from build123d import *

# Parameters (mm, degrees)
F0_R     = 12.7
F0_R_2   = 6.35
F1_DEPTH = 25.4
F2_R     = 5.08


with BuildPart() as f1:
    # F0 (on Front) → F1 (new body)
    with BuildSketch(Plane.XZ):
        Polygon((-25.4, 0), (0, 0), (25.4, 0), (25.4, 76.2), (63.5, 76.2), (63.5, 127), (-63.5, 127), (-63.5, 76.2), (-25.4, 76.2), align=None)
        with Locations((-38.1, 101.6)):
            Circle(F0_R, mode=Mode.SUBTRACT)
        with Locations((38.1, 101.6)):
            Circle(F0_R, mode=Mode.SUBTRACT)
        Polygon((25.4, 0), (0, 0), (-25.4, 0), (-25.4, -38.1), (-101.6, -38.1), (-101.6, -101.6), (101.6, -101.6), (101.6, -38.1), (25.4, -38.1), align=None)
        with Locations((-76.2, -69.85)):
            Circle(F0_R_2, mode=Mode.SUBTRACT)
        with Locations((-38.1, -69.85)):
            Circle(F0_R_2, mode=Mode.SUBTRACT)
        with Locations((38.1, -69.85)):
            Circle(F0_R_2, mode=Mode.SUBTRACT)
        with Locations((76.2, -69.85)):
            Circle(F0_R_2, mode=Mode.SUBTRACT)
    extrude(amount=F1_DEPTH)

    # F2
    f2_edges = [f1.edges().sort_by_distance(p)[0] for p in [
        (-25.4, -12.7, 76.2),
        (-25.4, -12.7, -38.1),
        (25.4, -12.7, -38.1),
        (25.4, -12.7, 76.2),
    ]]
    fillet(f2_edges, radius=F2_R)


solid = f1.part
The listing builds one solid part. Answer for the finished solid, in the listing's coordinates (mm). A direction names the side the tool comes from. Coordinates: 2 decimals unless noted, no trailing zeros. Write each loop counter-clockwise with the first axis right and the second up, starting at its lowest first coordinate (ties: lowest second). Pieces come first, ordered by that corner, then holes. Notation, with made-up numbers: (23, -11) -> (42, -11) arc R9 cw to (42, -5) -> close; hole circle Ø4 at (18, 6.25). An arc over 180 degrees is marked (long way). One line per question, with ' | ' between items.
1. For a pull along Z with two mould halves and no side action, classify faces 4 (the flat face through (-1, -13, -101.6)), 5 (the cylindrical face through (-39.753, -12.522, 114.192)), 6 (the flat face through (-1, -25.4, -11)) as released by +Z, released by -Z, zero draft, split by the parting line, or undercut.
Verdict:
face 4: released by -Z | face 5: undercut | face 6: zero draft
2. Section D-D (y = -11.5) is taken. Determine the outline of the cut face in (x, z).
Verdict:
outline: (-101.6, -101.6) -> (101.6, -101.6) -> (101.6, -38.1) -> (30.48, -38.1) arc R5.08 cw to (25.4, -33.02) -> (25.4, 71.12) arc R5.08 cw to (30.48, 76.2) -> (63.5, 76.2) -> (63.5, 127) -> (-63.5, 127) -> (-63.5, 76.2) -> (-30.48, 76.2) arc R5.08 cw to (-25.4, 71.12) -> (-25.4, -33.02) arc R5.08 cw to (-30.48, -38.1) -> (-101.6, -38.1) -> close; hole circle Ø12.7 at (-76.2, -69.85); hole circle Ø25.4 at (-38.1, 101.6); hole circle Ø12.7 at (-38.1, -69.85); hole circle Ø25.4 at (38.1, 101.6); hole circle Ø12.7 at (38.1, -69.85); hole circle Ø12.7 at (76.2, -69.85)
3. Given pin 1 Ø7.5 at (y, z) = (-16.5, 17.5) entering from +X; pin 2 Ø1 at (y, z) = (-15.5, 104) entering from +X; pin 3 Ø10 at (y, z) = (-5.5, 54.5) entering from -X, each flat-ended and moving along its own axis, determine where each tip first touches the part or whether it passes through.
Verdict:
pin 1: stops at x = 25.4 | pin 2: stops at x = 63.5 | pin 3: stops at x = -25.4
4. Which of the six approach directions +Z, -Z, +X, -X, +Y, -Y give full straight-line access (tool end or side, diameter ignored) to faces 1 (the flat face through (-25.4, -13, 20)), 2 (the flat face through (-63.5, -13, 102)), 3 (the flat face through (47, -13, 76.2))?
Verdict:
face 1: -X, +Y, -Y | face 2: +Z, -X, +Y, -Y | face 3: +X, +Y, -Y
5. Section B-B (z = 101.6) is taken. Determine the outline of the cut face in (x, y).
Verdict:
outline: (-63.5, -25.4) -> (-50.8, -25.4) -> (-50.8, 0) -> (-63.5, 0) -> close; (-25.4, -25.4) -> (25.4, -25.4) -> (25.4, 0) -> (-25.4, 0) -> close; (50.8, -25.4) -> (63.5, -25.4) -> (63.5, 0) -> (50.8, 0) -> close
6. Section A-A (x = 76.2) is taken. Determine the outline of the cut face in (y, z).
Verdict:
outline: (-25.4, -101.6) -> (0, -101.6) -> (0, -76.2) -> (-25.4, -76.2) -> close; (-25.4, -63.5) -> (0, -63.5) -> (0, -38.1) -> (-25.4, -38.1) -> close
7. Section C-C (x = -38.1) is taken. Determine the outline of the cut face in (y, z).
Verdict:
outline: (-25.4, -101.6) -> (0, -101.6) -> (0, -76.2) -> (-25.4, -76.2) -> close; (-25.4, -63.5) -> (0, -63.5) -> (0, -38.1) -> (-25.4, -38.1) -> close; (-25.4, 76.2) -> (0, 76.2) -> (0, 88.9) -> (-25.4, 88.9) -> close; (-25.4, 114.3) -> (0, 114.3) -> (0, 127) -> (-25.4, 127) -> close
8. Straight lines are drawn through the part: line 1 (Z direction, x = 38.1, y = -9.5); line 2 (Z direction, x = -62, y = -8.75); line 3 (X direction, y = -21.5, z = 92.5). For each, find the intervals that lie inside material, in ascending order.
Verdict:
line 1: z = -101.6 to -76.2, -63.5 to -38.1, 76.2 to 88.9, 114.3 to 127 | line 2: z = -101.6 to -38.1, 76.2 to 127 | line 3: x = -63.5 to -46.96, -29.24 to 29.24, 46.96 to 63.5
